from build123d import *

# Parameters (mm, degrees)
F0_R     = 10
F1_DEPTH = 10
F2_R     = 5
F3_DEPTH = 15
F4_DEPTH = 10


with BuildPart() as f1:
    # F0 (on Top) → F1 (new body)
    with BuildSketch(Plane.XY):
        Circle(F0_R)
    extrude(amount=F1_DEPTH)

    # F2 (on Top) → F3 (join)
    with BuildSketch(Plane.XY):
        Circle(F2_R)
    extrude(amount=F3_DEPTH)

    # F2 (on Top) → F4 (join)
    with BuildSketch(Plane.XY):
        Circle(F2_R)
    extrude(amount=-F4_DEPTH)


solid = f1.part
Source: CAD feature listing. Evaluate the final solid. Frame: model axes, mm. A direction names the side the tool comes from. Give positions to 0.01 mm unless a question says otherwise; leave off trailing zeros. Write each loop counter-clockwise with the first axis right and the second up, starting at its lowest first coordinate (ties: lowest second). Pieces come first, ordered by that corner, then holes. Notation, with made-up numbers: (2, 22.25) -> (50, 22.25) arc R23 cw to (50, 46.25) -> close; hole circle Ø9 at (40.25, 82.5). An arc over 180 degrees is marked (long way). Write item = value, one per line.
Q1. Cut plane D-D on z = 9. Return loops of the section in (x, y).
Here are the results:
outline = circle Ø20 at (0, 0)
Q2. Line query: line 1 (Z direction, x = -4.5, y = -2.75); line 2 (Y direction, x = 0, z = 2.75); line 3 (X direction, y = 0.25, z = -6.25). Output: solid intervals per line, ascending. Write a range as from..to.
Here are the results:
line_1 = 0..10
line_2 = -10..10
line_3 = -4.99..4.99
Q3. Cut plane C-C on z = -7.5. Return loops of the section in (x, y).
Here are the results:
outline = circle Ø10 at (0, 0)
Q4. First-contact query: pin 1 (1.5 mm diameter, centred on y = -7, z = 10, fed in from -X); pin 2 (2 mm diameter, centred on y = -5.5, z = 10.5, fed in from +X); pin 3 (6 mm diameter, centred on x = 6, z = 6, fed in from +Y). Flat tips, straight axial feed; report the tip coordinate or a pass-through.
Here are the results:
pin_1 = -7.81
pin_2 = 8.86
pin_3 = 9.54
Q5. Cut plane A-A on x = 0. Return loops of the section in (y, z), then the cut area to 3 significant figures.
Here are the results:
outline = (-10, 0) -> (-5, 0) -> (-5, -10) -> (5, -10) -> (5, 0) -> (10, 0) -> (10, 10) -> (5, 10) -> (5, 15) -> (-5, 15) -> (-5, 10) -> (-10, 10) -> close
area = 350 mm²
Q6. Reachability of faces 1 (the face through (-5, -2, 10)), 2 (the face through (-1.08, -4.88, -4.93)), 3 (the face through (0, 0, -10)) from +Z, -Z, +X, -X, +Y, -Y: full face, straight path, thin tool, end or side. Return the list, or none.
Here are the results:
face_1 = +Z
face_2 = -Z
face_3 = -Z, +X, -X, +Y, -Y
